Geometry check sheet. Reference: the model listing, model coordinates, mm. A direction names the side the tool comes from. Coordinates: 2 decimals unless noted, no trailing zeros. Answer as a JSON object with one key per item and string values. Group by question number.
from build123d import *


# Not quite as in the source:
# - a feature names something its author has since deleted; it is built from what else it names


with BuildPart() as f1:
    # F0 (on Front) → F1 (revolve)
    with BuildSketch(Plane.XZ):
        with BuildLine():
            Line((0, 47.625), (0, 21.59))
            Line((0, 21.59), (1.6002, 21.59))
            Line((1.6002, 21.59), (1.6002, 0.6053799298))
            Line((1.6002, 0.6053799298), (27.7014960486, 10.4798960957))
            ThreePointArc((27.7014960486, 10.4798960957), (30.6836253917, 12.8163260486), (31.8045894836, 16.435088247))
            Line((31.8045894836, 16.435088247), (31.7563839592, 35.5664000652))
            ThreePointArc((31.7563839592, 35.5664000652), (31.0101790546, 37.3583125654), (29.2163920223, 38.1))
            Line((29.2163920223, 38.1), (7.62, 38.1))
            Line((7.62, 38.1), (7.62, 57.15))
            Line((7.62, 57.15), (4.7625, 57.15))
            Line((4.7625, 57.15), (4.7625, 47.625))
            Line((4.7625, 47.625), (0, 47.625))
        make_face()
    revolve(axis=Axis((0, 0, 28.575), (0, 0, 1)))


solid = f1.part
(1) Gauge pin test, flat ends, axial feed: pin 1 (10.5 mm diameter, centred on x = -1, y = 1.5, fed in from +Z); pin 2 (10 mm diameter, centred on y = -24.5, z = 37, fed in from -X); pin 3 (8 mm diameter, centred on x = -22, y = -5.5, fed in from +Z); pin 4 (2 mm diameter, centred on y = 9, z = 39.5, fed in from +X). Record the tip position at first contact, or that the pin passes through.
(2) Set-up check for faces 1 (the face through (-1.27, -0.974, 10.951)), 2 (the face through (0, -5, 57.15)): record each of +Z, -Z, +X, -X, +Y, -Y from which the full face is reachable in a straight line by a thin tool's end or side.
(3) Draft check along Y on faces 3 (the face through (6, -6, 38.1)), 4 (the face through (0, 0, 47.625)), 5 (the face through (-1.65, -7.44, 47.76)), 6 (the face through (-3.78, -2.9, 52.32)). Enter one of: +Y half, -Y half, draft (parallel to the pull), parting line (faces both ways), or undercut.
(4) Material ranges on L1, parallel to Y at x = 0, z = 14; L2, parallel to Y at x = 0, z = 11.25; L3, parallel to Y at x = -1.5, z = 29, recorded low to high. Write a range as [from, to].
Conclusion:
{
 "1": {"pin 1": "stops at z = 57.15", "pin 2": "stops at x = -24.94", "pin 3": "stops at z = 38.1", "pin 4": "passes through"},
 "2": {"face 1": "-Z", "face 2": "+Z, +X, -X, +Y, -Y"},
 "3": {"face 3": "draft", "face 4": "undercut", "face 5": "parting line", "face 6": "undercut"},
 "4": {"L1": "y = [-31.33, -1.6], [1.6, 31.33]", "L2": "y = [-29.14, -1.6], [1.6, 29.14]", "L3": "y = [-31.74, 31.74]"}
}
